The model under review builds one solid part; all positions refer to its coordinate system, in mm. A direction names the side the tool comes from. Give positions to 0.01 mm unless a question says otherwise; leave off trailing zeros. Loops run counter-clockwise (first coordinate to the right, second up) from the corner with the lowest first, then second, coordinate; pieces in that order, holes last. Notation, with made-up numbers: M 80.5,-23.5 L 126.5,-23.5 A13 cw 126.5,-5.5 Z; hole C 32,50 d10. An arc over 180 degrees is marked long. Write item = value, one per line. Start each with the question number.
1. We need section B-B on x = 33. Give the boundary of the cut face in (y, z), then the cut area to 3 significant figures.
2. We need section A-A on y = 6. Give the boundary of the cut face in (x, z), then the cut area to 3 significant figures.
3. We need section C-C on y = 24. Give the boundary of the cut face in (x, z), then the cut area to 3 significant figures.
4. For faces 5 (the face through (17, 0, 3)), 6 (the face through (9, 5, 3)), 7 (the face through (14.75, 3, 3)), list the 3-axis set-ups (+Z, -Z, +X, -X, +Y, -Y) from which the entire face can be reached by the end or side of a thin tool; tool diameter is ignored.
5. For pin 1 (1 mm diameter, centred on x = 4, z = 2.5, fed in from -Y); pin 2 (1.8 mm diameter, centred on y = 10.5, z = 3.5, fed in from -X); pin 3 (2 mm diameter, centred on x = 30.5, z = 4.5, fed in from +Y), all flat-tipped, find the tip position at first contact; note any pin that passes through.
6. Wall thickness on line 1 along X through (y, z) = (0.5, 1.2); line 2 along X through (y, z) = (-3, 4.05); line 3 along Y through (x, z) = (7.5, 5.5): over which ranges is each line inside the solid? List them lowest first. Write a range as from..to.
7. Draft analysis for pull direction X (two halves, no side actions). For faces 1 (the face through (-4.413, 8.519, 3.042)), 2 (the face through (74, 0, 3)), 3 (the face through (62.57, -5.4, 3.04)), 4 (the face through (78, 4, 3)), state which applies: pulls with the +X half, pulls with the -X half, needs draft (parallel to the pull), parting line crosses it, or undercut.
Autodesk Inventor part; units mm, degrees
ref_plane "YZ Plane" through (0, 0, 0) normal (1, 0, 0) x (0, 1, 0)
ref_plane "XZ Plane" through (0, 0, 0) normal (0, 1, 0) x (-1, 0, 0)
ref_plane "XY Plane" through (0, 0, 0) normal (0, 0, 1) x (1, 0, 0)
sketch "Sketch1" plane through (0, 0, 0) normal (0, 0, 1) x (1, 0, 0)
  line L0 (0, 29) -> (0, 0)
  line L1 (0, 0) -> (78, 0)
  line L2 (78, 0) -> (78, 8)
  line L3 (78, 8) -> (4, 29)
  line L4 (4, 29) -> (0, 29)
  dimension "d0" = 29
  dimension "d1" = 78
  dimension "d2" = 4
  dimension "d3" = 8
extrude "Extrusion1" add sketch "Sketch1" along normal blind 6
sketch "Sketch2" plane through (0, 0, 6) normal (0, 0, 1) x (1, 0, 0)
  line L0 (0, 29) -> (0, 0)
  line L1 (0, 0) -> (78, 0)
  line L2 (78, 0) -> (78, 8)
  line L3 (4, 29) -> (0, 29)
  circle A0 centre (-11.099, 13.5) radius 7.5 construction
  line L4 (-6, 19) -> (-6, 8) construction
  arc A1 (-4.396, 9.5114) -> (-4.396, 17.4886) centre (-11.099, 13.5) ccw
  line L5 (-3.5366, 19) -> (0, 19)
  line L6 (-3.5366, 8) -> (0, 8)
  arc A2 (-3.5366, 19) -> (-4.396, 17.4886) centre (-3.5366, 18) ccw
  arc A3 (-4.396, 9.5114) -> (-3.5366, 8) centre (-3.5366, 9) ccw
  line L7 (20, 0) -> (28, 0)
  line L8 (28, 0) -> (28, -4)
  line L9 (26, -6) -> (22, -6)
  line L10 (20, -4) -> (20, 0)
  line L11 (62, 0) -> (70, 0)
  line L12 (70, 0) -> (70, -4)
  line L13 (68, -6) -> (64, -6)
  line L14 (62, -4) -> (62, 0)
  arc A4 (20, -4) -> (22, -6) centre (22, -4) ccw
  arc A5 (26, -6) -> (28, -4) centre (26, -4) ccw
  arc A6 (62, -4) -> (64, -6) centre (64, -4) ccw
  arc A7 (68, -6) -> (70, -4) centre (68, -4) ccw
  point P0 (-5.5682, 19)
  point P1 (-5.5682, 8)
  dimension "d6" = 15
  dimension "d7" = 11
  dimension "d8" = 6
  dimension "d9" = 11
  dimension "d10" = 7.8
  dimension "d11" = 10
  dimension "d12" = 1
  dimension "d13" = 2
  dimension "d15" = 8
  dimension "d17" = 8
  dimension "d18" = 6
  dimension "d19" = 20
  dimension "d20" = 8
extrude "Extrusion2" add sketch "Sketch2" against normal blind 6
sketch "Sketch3" plane through (0, 0, 6) normal (0, 0, 1) x (1, 0, 0)
  line L0 (0, 0) -> (20, 0)
  line L1 (20, 0) -> (20, -4)
  line L2 (10.25, 16.3) -> (14.75, 16.3)
  line L3 (14.75, 0) -> (10.25, 0)
  line L4 (17.25, 12.3) -> (17.25, 5)
  line L5 (7.75, 5) -> (7.75, 12.3)
  line L6 (7.75, 12.3) -> (10.25, 12.3)
  line L7 (14.75, 12.3) -> (17.25, 12.3)
  line L8 (17.25, 5) -> (14.75, 5)
  line L9 (10.25, 5) -> (7.75, 5)
  line L10 (10.25, 0) -> (10.25, 5)
  line L11 (10.25, 12.3) -> (10.25, 16.3)
  line L12 (14.75, 16.3) -> (14.75, 12.3)
  line L13 (14.75, 5) -> (14.75, 0)
  point P0 (12.5, 16.3)
  dimension "d23" = 4.5
  dimension "d24" = 2.5
  dimension "d25" = 2.5
  dimension "d26" = 4
  dimension "d27" = 5
  dimension "d28" = 7.3
  dimension "d29" = 7.5
extrude "Extrusion3" cut sketch "Sketch3" against normal through all
properties part number "x_carryage_brace"
Final values:
q1.outline = M 0,0 L 20.77,0 L 20.77,6 L 0,6 Z
q1.area = 125 mm²
q2.outline = M 0,0 L 7.75,0 L 7.75,6 L 0,6 Z; M 17.25,0 L 78,0 L 78,6 L 17.25,6 Z
q2.area = 411 mm²
q3.outline = M 0,0 L 21.62,0 L 21.62,6 L 0,6 Z
q3.area = 130 mm²
q4.face_5 = +Z, -Z, -X, -Y
q4.face_6 = +Z, -Z
q4.face_7 = +Z, -Z, -Y
q5.pin_1 = 0
q5.pin_2 = -4.34
q5.pin_3 = 21.76
q6.line_1 = 0..10.25, 14.75..78
q6.line_2 = 20..28, 62..70
q6.line_3 = 0..28.01
q7.face_1 = pulls with the -X half
q7.face_2 = needs draft
q7.face_3 = undercut
q7.face_4 = pulls with the +X half
